Could you check a few things on this model? Use its own coordinates, in mm. Face numbers are marked on the shaded views. A direction names the side the tool comes from. Round coordinates to 2 decimals unless told otherwise and drop trailing zeros. Loops run counter-clockwise (first coordinate to the right, second up) from the corner with the lowest first, then second, coordinate; pieces in that order, holes last.
from build123d import *

# Parameters (mm, degrees)
SKETCH1_R           = 7.0485
BOSS_EXTRUDE1_DEPTH = 0.4953
SKETCH2_R           = 4.8514
BOSS_EXTRUDE2_DEPTH = 4.064
SKETCH3_R           = 7.0485
BOSS_EXTRUDE3_DEPTH = 0.4953
SKETCH4_R           = 7.0485
BOSS_EXTRUDE4_DEPTH = 6.0198
SKETCH5_R           = 2.38125
CUT_EXTRUDE1_DEPTH  = 12.0744


with BuildPart() as part:
    # Sketch1 → Boss-Extrude1 (new body)
    with BuildSketch(Plane(origin=(0, 0, 0), x_dir=(0, 0, -1), z_dir=(1, 0, 0))):
        Circle(SKETCH1_R)
    extrude(amount=BOSS_EXTRUDE1_DEPTH)

    # Sketch2 → Boss-Extrude2 (add)
    with BuildSketch(Plane(origin=(0.4953, 0, 0), x_dir=(0, 0, -1), z_dir=(1, 0, 0))):
        Circle(SKETCH2_R)
    extrude(amount=BOSS_EXTRUDE2_DEPTH)

    # Sketch3 → Boss-Extrude3 (add)
    with BuildSketch(Plane(origin=(4.5593, 0, 0), x_dir=(0, 0, -1), z_dir=(1, 0, 0))):
        Circle(SKETCH3_R)
    extrude(amount=BOSS_EXTRUDE3_DEPTH)

    # Sketch4 → Boss-Extrude4 (add)
    with BuildSketch(Plane(origin=(5.0546, 0, 0), x_dir=(0, 0, -1), z_dir=(1, 0, 0))):
        Circle(SKETCH4_R)
    extrude(amount=BOSS_EXTRUDE4_DEPTH)

    # Sketch5 → Cut-Extrude1 (cut, through all)
    with BuildSketch(Plane(origin=(11.0744, 0, 0), x_dir=(0, 0, -1), z_dir=(1, 0, 0))):
        Circle(SKETCH5_R)
    extrude(amount=-CUT_EXTRUDE1_DEPTH, mode=Mode.SUBTRACT)


solid = part.part
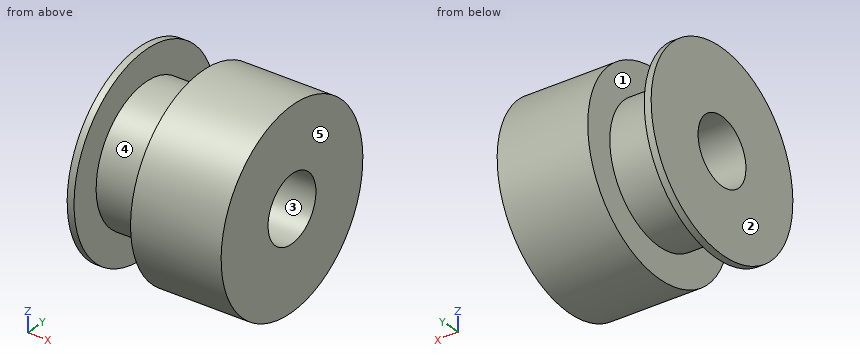
Item 1: If we section it at A-A, the plane z = 0: Please give me the cut outline in (x, y).
Results list:
outline: (0, -7.05) - (0.5, -7.05) - (0.5, -4.85) - (4.56, -4.85) - (4.56, -7.05) - (11.07, -7.05) - (11.07, -2.38) - (0, -2.38) - close; (0, 2.38) - (11.07, 2.38) - (11.07, 7.05) - (4.56, 7.05) - (4.56, 4.85) - (0.5, 4.85) - (0.5, 7.05) - (0, 7.05) - close
Item 2: If we section it at C-C, the plane x = 10: Please give me the cut outline in (y, z).
Results list:
outline: circle Ø14.1 at (0, 0); hole circle Ø4.76 at (0, 0)
Item 3: Will these pins go through, and if not, where does the flat tip stop? pin 1 (3 mm diameter, centred on y = 3, z = -2, fed in from -X); pin 2 (5 mm diameter, centred on x = 3.5, y = 3, fed in from +Z); pin 3 (3 mm diameter, centred on x = 4.5, z = -4.5, fed in from -Y); pin 4 (2 mm diameter, centred on x = 5, z = -3.5, fed in from +Y).
Results list:
pin 1: stops at x = 0
pin 2: stops at z = 7.01
pin 3: stops at y = -6.38
pin 4: stops at y = 6.59
Item 4: If I drill on line 1 along X through (y, z) = (3.75, 5.75); line 2 along Y through (x, z) = (6.5, 0); line 3 along Z through (x, y) = (10.25, -0.75), over which ranges is the centre line in solid material (lowest first)?
Results list:
line 1: x = 0 to 0.5, 4.56 to 11.07
line 2: y = -7.05 to -2.38, 2.38 to 7.05
line 3: z = -7.01 to -2.26, 2.26 to 7.01
Item 5: For the marked faces 1 and 2, which set-ups out of +Z, -Z, +X, -X, +Y, -Y let a thin tool reach every point of the face, with its end or its side?
Results list:
face 1: none
face 2: +Z, -Z, -X, +Y, -Y
Item 6: We'd pull the mould along Z, two halves only. Please class the marked faces 3, 4 and 5: released by +Z, released by -Z, zero draft, split by the parting line, or undercut.
Results list:
face 3: undercut
face 4: split by the parting line
face 5: zero draft
Item 7: If we section it at D-D, the plane y = 6.25: Please give me the cut outline in (x, z).
Results list:
outline: (0, -3.26) - (0.5, -3.26) - (0.5, 3.26) - (0, 3.26) - close; (4.56, -3.26) - (11.07, -3.26) - (11.07, 3.26) - (4.56, 3.26) - close
